Could you check a few things on this model? Use its own coordinates, in mm. Give positions to 0.01 mm unless a question says otherwise; leave off trailing zeros. Write each loop counter-clockwise with the first axis right and the second up, starting at its lowest first coordinate (ties: lowest second). Pieces come first, ordered by that corner, then holes. Notation, with made-up numbers: M -1.5,21.25 L 44.5,21.25 A13 cw 44.5,25.25 Z; hole C -31,-6.5 d4. An arc over 180 degrees is marked long. One line per item, written item: value.
Autodesk Inventor part; units mm, degrees
ref_plane "YZ Plane" through (0, 0, 0) normal (1, 0, 0) x (0, 1, 0)
ref_plane "XZ Plane" through (0, 0, 0) normal (0, 1, 0) x (-1, 0, 0)
ref_plane "XY Plane" through (0, 0, 0) normal (0, 0, 1) x (1, 0, 0)
sketch "Sketch1" plane through (0, 0, 0) normal (0, 0, 1) x (1, 0, 0)
  circle A0 centre (0, 0) radius 3.5
  circle A1 centre (43.8036, 0) radius 3.5
  line L0 (-20.2073, 0) -> (-10.1036, 17.5)
  line L1 (-10.1036, 17.5) -> (10.1036, 17.5)
  line L2 (10.1036, 17.5) -> (20.2073, 0)
  line L3 (20.2073, 0) -> (10.1036, -17.5)
  line L4 (10.1036, -17.5) -> (-10.1036, -17.5)
  line L5 (-10.1036, -17.5) -> (-20.2073, 0)
  line L6 (64.0108, 0) -> (53.9072, -17.5)
  line L7 (53.9072, -17.5) -> (33.6999, -17.5)
  line L8 (33.6999, -17.5) -> (23.5963, 0)
  line L9 (23.5963, 0) -> (33.6999, 17.5)
  line L10 (33.6999, 17.5) -> (53.9072, 17.5)
  line L11 (53.9072, 17.5) -> (64.0108, 0)
  line L12 (10.1036, 17.5) -> (33.6999, 17.5)
  line L13 (10.1036, -17.5) -> (33.6999, -17.5)
  dimension "d0" = 7
  dimension "d1" = 7
  dimension "d2" = 43.8036
  dimension "d3" = 35
extrude "Extrusion1" add sketch "Sketch1" along normal blind 4 contours A0 | L0 L1 L2 L3 L4 L5 | L12 L9 L8 L13 L3 L2 | L10 L11 L6 L7 L8 L9
sketch "Sketch2" plane through (0, 0, 4) normal (0, 0, 1) x (1, 0, 0)
  circle A0 centre (43.8036, 0) radius 3.5
  circle A1 centre (0, 0) radius 3.5
  line L0 (-10.1036, 17.5) -> (-20.2073, 0)
  line L1 (-20.2073, 0) -> (-10.1036, -17.5)
  line L2 (53.9072, -17.5) -> (64.0108, 0)
  line L3 (64.0108, 0) -> (53.9072, 17.5)
  line L4 (57.3713, 17.5) -> (67.4749, 0)
  line L5 (67.4749, 0) -> (57.3713, -17.5)
  line L6 (-13.5677, 17.5) -> (-23.6714, 0)
  line L7 (-23.6714, 0) -> (-13.5677, -17.5)
  line L8 (53.9072, 17.5) -> (-10.1036, 17.5)
  line L9 (-10.1036, 17.5) -> (-13.5677, 17.5)
  line L10 (-13.5677, -17.5) -> (-10.1036, -17.5)
  line L11 (-10.1036, -17.5) -> (53.9072, -17.5)
  line L12 (53.9072, -17.5) -> (57.3713, -17.5)
  line L13 (64.0108, 0) -> (53.9072, 17.5)
  line L14 (53.9072, 17.5) -> (57.3713, 17.5)
  point P0 (-11.8357, -17.5)
  dimension "d6" = 3
  dimension "d7" = 3
extrude "Extrusion2" add sketch "Sketch2" against normal up to surface (4 mm away) from surface at 0 contours L0 L1 L10 L7 L6 L9 | L14 L4 L5 L12 L2 L3
sketch "Sketch3" plane through (0, 0, 4) normal (0, 0, 1) x (1, 0, 0)
  circle A0 centre (-20.6714, 0) radius 1.25
  circle A1 centre (64.4749, 0) radius 1.25
  circle A2 centre (21.9018, 10) radius 1.25
  circle A3 centre (21.9018, -10) radius 1.25
  line L0 (21.9018, 10) -> (21.9018, -10)
  line L1 (-13.5677, 17.5) -> (57.3713, 17.5)
  line L2 (-20.6714, 0) -> (64.4749, 0)
  point P0 (0, 0)
  point P1 (21.9018, 17.5)
  point P2 (-10.1036, 17.5)
  point P3 (21.9018, 17.5)
  point P4 (21.9018, 0)
  dimension "d10" = 2.5
  dimension "d11" = 2.5
  dimension "d12" = 2.5
  dimension "d13" = 2.5
  dimension "d14" = 20
  dimension "d34" = 85.1463
extrude "Extrusion3" cut sketch "Sketch3" against normal through all
sketch "Sketch4" plane through (0, 0, 4) normal (0, 0, 1) x (1, 0, 0)
  line L0 (0, 8.5) -> (0, -8.5) construction
  line L1 (43.8036, 8.5) -> (43.8036, -8.5) construction
  circle A0 centre (43.8036, 0) radius 3.5 construction
  circle A1 centre (0, 0) radius 3.5 construction
  circle A2 centre (0, 8.5) radius 1.05
  circle A3 centre (0, -8.5) radius 1.05
  circle A4 centre (43.8036, -8.5) radius 1.05
  circle A5 centre (43.8036, 8.5) radius 1.05
  dimension "d19" = 17
  dimension "d20" = 17
  dimension "d21" = 2.1
  dimension "d22" = 2.1
  dimension "d23" = 2.1
  dimension "d24" = 2.1
extrude "Extrusion4" cut sketch "Sketch4" against normal through all
sketch "Sketch8" plane through (0, 0, 4) normal (0, 0, 1) x (1, 0, 0)
  circle A0 centre (-20.6714, 0) radius 1.25
  circle A1 centre (-20.6714, 0) radius 4.4214
  circle A2 centre (64.4749, 0) radius 1.25
  circle A3 centre (64.4749, 0) radius 4.4214
  point P0 (0, 0)
  dimension "d30" = 8.8427
  dimension "d31" = 8.8427
extrude "Extrusion5" add sketch "Sketch8" against normal up to surface (4 mm away) from surface at 0
sketch "Sketch9" plane through (0, 0, 0) normal (0, 0, -1) x (-1, 0, 0)
  line L0 (6.3509, 0) -> (3.1754, -5.5)
  line L1 (3.1754, -5.5) -> (-3.1754, -5.5)
  line L2 (-3.1754, -5.5) -> (-6.3509, 0)
  line L3 (-6.3509, 0) -> (-3.1754, 5.5)
  line L4 (-3.1754, 5.5) -> (3.1754, 5.5)
  line L5 (3.1754, 5.5) -> (6.3509, 0)
  circle A0 centre (-43.8036, 0) radius 3.5
  line L6 (-37.4527, 0) -> (-40.6281, -5.5)
  line L7 (-40.6281, -5.5) -> (-46.979, -5.5)
  line L8 (-46.979, -5.5) -> (-50.1544, 0)
  line L9 (-50.1544, 0) -> (-46.979, 5.5)
  line L10 (-46.979, 5.5) -> (-40.6281, 5.5)
  line L11 (-40.6281, 5.5) -> (-37.4527, 0)
  circle A1 centre (-43.8036, 0) radius 3.5
  circle A2 centre (0, 0) radius 3.5
  dimension "d35" = 11
  dimension "d36" = 11
extrude "Extrusion6" cut sketch "Sketch9" against normal blind 2 contours L0 L1 L2 L3 L4 L5 | A0 | L6 L7 L8 L9 L10 L11 | A2
sketch "Sketch10" plane through (0, 0, 0) normal (0, 0, -1) x (-1, 0, 0)
  line L0 (3.1754, 5.5) -> (6.3509, 0)
  circle A0 centre (0, 0) radius 6.3509
  circle A1 centre (-43.8036, 0) radius 3.5
  line L1 (-37.4527, 0) -> (-40.6281, -5.5)
  circle A2 centre (-43.8036, 0) radius 6.3509
extrude "Extrusion7" cut sketch "Sketch10" against normal through all contours A0 L0 | L0 A0 | A1 | A2 L1 | L1 A2
equation "\"d7\" = d6"
equation "\"d31\" = d30"
properties part number "AC09" material "ABS Plastic"
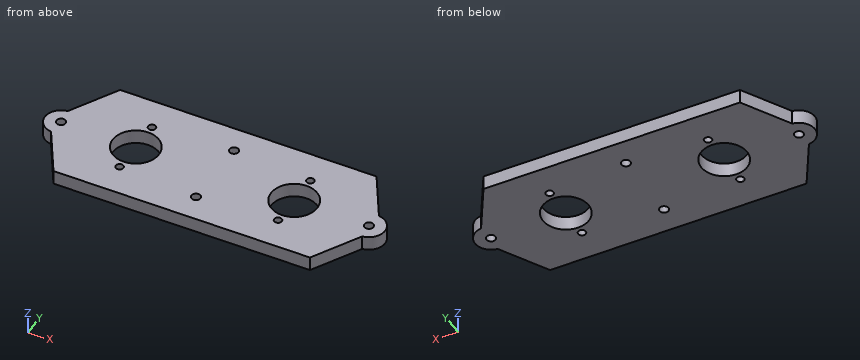
1) If we section it at A-A, the plane x = 0: Write out the boundary of the cut face in (y, z), then the cut area to 3 significant figures.
Outcome:
outline: M -17.5,0 L -9.55,0 L -9.55,4 L -17.5,4 Z; M -7.45,0 L -6.35,0 L -6.35,4 L -7.45,4 Z; M 6.35,0 L 7.45,0 L 7.45,4 L 6.35,4 Z; M 9.55,0 L 17.5,0 L 17.5,4 L 9.55,4 Z
area: 72.4 mm^2
2) If we section it at C-C, the plane z = 0.9: Give the number of separate pieces and of enclosed holes in the cut face, then the cut area to 3 significant figures.
Outcome:
separate pieces: 1
enclosed holes: 10
area: 2,580 mm^2
3) If we section it at B-B, the plane y = 0: Write out the boundary of the cut face in (x, z), then the cut area to 3 significant figures.
Outcome:
outline: M -25.09,0 L -21.92,0 L -21.92,4 L -25.09,4 Z; M -19.42,0 L -6.35,0 L -6.35,4 L -19.42,4 Z; M 6.35,0 L 37.45,0 L 37.45,4 L 6.35,4 Z; M 50.15,0 L 63.22,0 L 63.22,4 L 50.15,4 Z; M 65.72,0 L 68.9,0 L 68.9,4 L 65.72,4 Z
area: 254 mm^2
4) Please list where these lines run through material, in increasing order: L1, parallel to Y at x = 0, z = 1.5; L2, parallel to X at y = -1, z = 2.75; L3, parallel to X at y = 8, z = 1.9. Write a range as from..to.
Outcome:
L1: y = -17.5..-9.55, -7.45..-6.35, 6.35..7.45, 9.55..17.5
L2: x = -24.98..-21.42, -19.92..-6.27, 6.27..37.53, 50.08..63.72, 65.22..68.78
L3: x = -19.05..-0.92, 0.92..42.88, 44.73..62.86
5) If we section it at D-D, the plane y = 13: Write out the boundary of the cut face in (x, z).
Outcome:
outline: M -16.17,0 L 59.97,0 L 59.97,4 L -16.17,4 Z
